from build123d import *

# Parameters (mm, degrees)
SKETCH12_W          = 5
SKETCH12_H          = 20
BOSS_EXTRUDE3_DEPTH = 3
SKETCH13_R          = 10
BOSS_EXTRUDE4_DEPTH = 5
BOSS_EXTRUDE6_START = -5
SKETCH14_R          = 10
BOSS_EXTRUDE6_DEPTH = 5


with BuildPart() as part:
    # Sketch12 → Boss-Extrude3 (new body)
    with BuildSketch(Plane(origin=(0, 0, 0), x_dir=(1, 0, 0), z_dir=(0, 1, 0))):
        Polygon((7.992304902, 33.129302691), (0, 25.13699779), (0, 20), (5, 20), (5, 0), (45, 0), (45, 20), (50, 20), (50, 26.444694099), (43.315391407, 33.129302691), align=None)
        with Locations((47.5, 10)):
            Rectangle(SKETCH12_W, SKETCH12_H)
        with Locations((2.5, 10)):
            Rectangle(SKETCH12_W, SKETCH12_H)
    extrude(amount=BOSS_EXTRUDE3_DEPTH)

    # Sketch13 → Boss-Extrude4 (add)
    with BuildSketch(Plane.ZY):
        Circle(SKETCH13_R)
    extrude(amount=-BOSS_EXTRUDE4_DEPTH)

    # Sketch14 → Boss-Extrude6 (add)
    with BuildSketch(Plane(origin=(50, 0, 0), x_dir=(0, 0, -1), z_dir=(1, 0, 0)).offset(BOSS_EXTRUDE6_START)):
        Circle(SKETCH14_R)
    extrude(amount=BOSS_EXTRUDE6_DEPTH)


solid = part.part
Input: part model. Units: mm. Frame: model coordinates. A direction names the side the tool comes from. Give positions to 0.01 mm unless a question says otherwise; leave off trailing zeros. Order: outer loops, then holes, each group sorted by start corner. A loop starts at its lowest first (then second) coordinate and runs counter-clockwise, first axis right, second up.
Q1. Section D-D on z = -6.5. Output: boundary loops of the cut face in (x, y), and give its area (3 significant figures).
Checked values:
outline: (0, -7.6) - (5, -7.6) - (5, 0) - (45, 0) - (45, -7.6) - (50, -7.6) - (50, 7.6) - (45, 7.6) - (45, 3) - (5, 3) - (5, 7.6) - (0, 7.6) - close
area: 272 mm2
Q2. Contact query for flat-ended pins moving along their axis: pin 1 Ø0.9 at (x, y) = (15.5, 1.5) entering from +Z; pin 2 Ø10 at (x, y) = (7.5, -5.5) entering from -Z; pin 3 Ø4 at (x, z) = (18.5, -16.5) entering from -Y. Output: stop coordinate, or through.
Checked values:
pin 1: stops at z = 0
pin 2: stops at z = -9.93
pin 3: stops at y = 0
Q3. Set-up query: faces 1 (the flat face through (5, 0, 2)), 2 (the flat face through (25, 0, -17)), 3 (the flat face through (25, 1, 0)). Return all of +Z, -Z, +X, -X, +Y, -Y with unobstructed straight access to the full face (end or side cutting, diameter ignored); none if empty.
Checked values:
face 1: +Z
face 2: -Z, -Y
face 3: +Z, +Y, -Y
Q4. Draft query along X for faces 4 (the flat face through (25, 3, -17)), 5 (the flat face through (4.052, 1.479, -29.189)), 6 (the flat face through (26, 1, -33.129)). Return one class per face: +X half, -X half, draft (parallel to the pull), parting line (faces both ways), or undercut.
Checked values:
face 4: undercut
face 5: -X half
face 6: draft
Q5. Section B-B on z = 4. Output: boundary loops of the cut face in (x, y).
Checked values:
outline: (0, -9.17) - (5, -9.17) - (5, 9.17) - (0, 9.17) - close; (45, -9.17) - (50, -9.17) - (50, 9.17) - (45, 9.17) - close
Q6. Ray query, probe 1 along X at (y, z) = (3.25, -7); probe 2 along Y at (x, z) = (24, -25); probe 3 along Y at (x, z) = (45.5, 5.5). Return the intervals inside material, ascending.
Checked values:
probe 1: x = 0 to 5, 45 to 50
probe 2: y = 0 to 3
probe 3: y = -8.35 to 8.35
Q7. Section A-A on y = -5.25. Output: boundary loops of the cut face in (x, z).
Checked values:
outline: (0, -8.51) - (5, -8.51) - (5, 8.51) - (0, 8.51) - close; (45, -8.51) - (50, -8.51) - (50, 8.51) - (45, 8.51) - close
Q8. Section C-C on y = 1. Output: boundary loops of the cut face in (x, z), and give its area (3 significant figures).
Checked values:
outline: (0, -25.14) - (7.99, -33.13) - (43.32, -33.13) - (50, -26.44) - (50, 9.95) - (45, 9.95) - (45, 0) - (5, 0) - (5, 9.95) - (0, 9.95) - close
area: 1,700 mm2
